Drawing for the job (mm, zero at the part's lowest x, y, z). A direction names the side the tool comes from. Give positions to 0.01 mm unless a question says otherwise; leave off trailing zeros. Write each loop counter-clockwise with the first axis right and the second up, starting at its lowest first coordinate (ties: lowest second). Pieces come first, ordered by that corner, then holes. Notation, with made-up numbers: M -5,-22.75 L 0,-22.75 A28 ccw 0,9.25 Z; hole C -9.75,17.25 d7. An arc over 180 degrees is marked long. Answer as a JSON object with one key per item and string values. Group by question number.
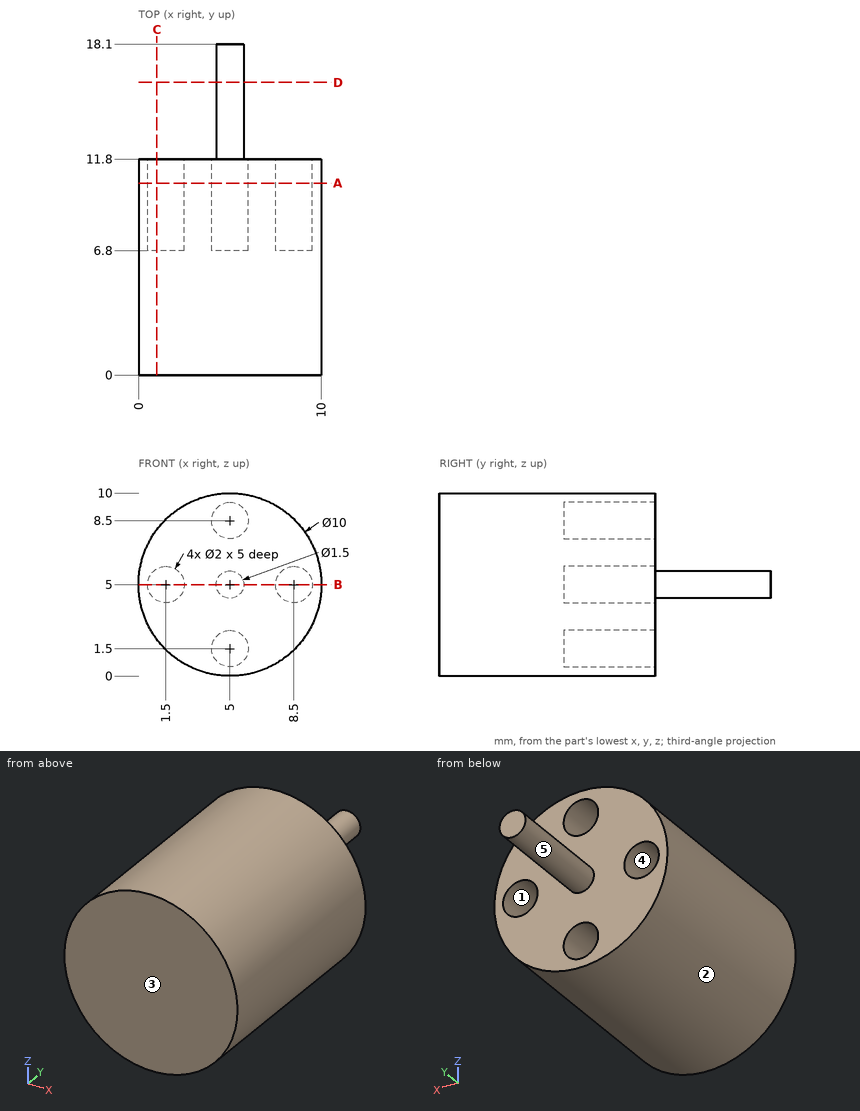
Q1. 3-axis set-ups, long thin cutter, end or side, ignore diameter. For the marked faces 1 and 2: which of +Z, -Z, +X, -X, +Y, -Y reach the whole face in a straight line?
Q2. Slice it at B-B, the plane z = 5. Write the cut outline in (x, y).
Q3. Two-plate mould, pull along Z, no slides. Class the marked faces 3, 4 and 5: +Z half, -Z half, draft (parallel to the pull), parting line (faces both ways), or undercut.
Q4. Wall check: L1, parallel to X at y = 8.2, z = 5; L2, parallel to Y at x = 9, z = 4.75; L3, parallel to Z at x = 4.25, y = 7.5. Give the ranges that are in metal, low to high.
Q5. Slice it at A-A, the plane y = 10.5. Write the cut outline in (x, z), then the cut area to 3 significant figures.
Q6. Slice it at D-D, the plane y = 16. Write the cut outline in (x, z), then the cut area to 3 significant figures.
Q7. Slice it at C-C, the plane x = 1. Write the cut outline in (y, z), then the cut area to 3 significant figures.
Q8. Drop flat-ended pins along their axis: P1, Ø1.5, axis at x = 1.5, y = 12, coming from the -Z side; P2, Ø1.2, axis at x = 5, z = 1.5, coming from the +Y side; P3, Ø2, axis at x = 5, z = 2, coming from the +Y side. Give the stop position or say it passes through.
Solved:
{
 "1": {"face 1": "+Y", "face 2": "+Y, -Y"},
 "2": {"outline": "M 0,0 L 10,0 L 10,11.8 L 9.5,11.8 L 9.5,6.8 L 7.5,6.8 L 7.5,11.8 L 5.75,11.8 L 5.75,18.1 L 4.25,18.1 L 4.25,11.8 L 2.5,11.8 L 2.5,6.8 L 0.5,6.8 L 0.5,11.8 L 0,11.8 Z"},
 "3": {"face 3": "draft", "face 4": "undercut", "face 5": "parting line"},
 "4": {"L1": "x = 0 to 0.5, 2.5 to 7.5, 9.5 to 10", "L2": "y = 0 to 6.8", "L3": "z = 0.06 to 0.84, 2.16 to 7.84, 9.16 to 9.94"},
 "5": {"outline": "C 5,5 d10; hole C 1.5,5 d2; hole C 5,1.5 d2; hole C 5,8.5 d2; hole C 8.5,5 d2", "area": "66.0 mm²"},
 "6": {"outline": "C 5,5 d1.5", "area": "1.77 mm²"},
 "7": {"outline": "M 0,2 L 11.8,2 L 11.8,4.13 L 6.8,4.13 L 6.8,5.87 L 11.8,5.87 L 11.8,8 L 0,8 Z", "area": "62.1 mm²"},
 "8": {"P1": "stops at z = 0.84", "P2": "stops at y = 6.8", "P3": "stops at y = 11.8"}
}
